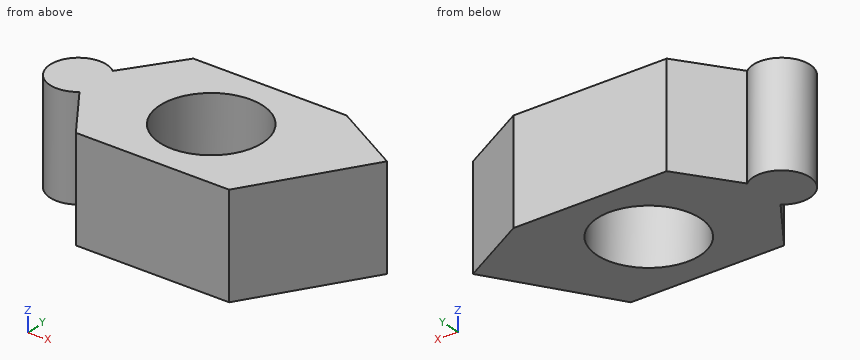
from build123d import *

# Parameters (mm, degrees)
F0_W     = 15
F0_H     = 15
F0_R     = 5
F1_DEPTH = 5
F3_DEPTH = 5
F5_DEPTH = 5


with BuildPart() as f1:
    # F0 (on Top) → F1 (new body, symmetric)
    with BuildSketch(Plane.XY):
        Rectangle(F0_W, F0_H)
        Circle(F0_R, mode=Mode.SUBTRACT)
    extrude(amount=F1_DEPTH, both=True)

    # F2 (on Top) → F3 (join, symmetric)
    with BuildSketch(Plane.XY):
        with BuildLine():
            Line((-7.5, 7.5), (-11.260282, 2.129761))
            ThreePointArc((-11.260282, 2.129761), (-15.75, 0), (-11.260282, -2.129761))
            Line((-11.260282, -2.129761), (-7.5, -7.5))
            Line((-7.5, -7.5), (-7.5, 7.5))
        make_face()
    extrude(amount=F3_DEPTH, both=True)

    # F4 (on Top) → F5 (join, symmetric)
    with BuildSketch(Plane.XY):
        Polygon((14.467447, 3.568756), (7.5, 7.5), (7.5, -7.5), align=None)
    extrude(amount=F5_DEPTH, both=True)


solid = f1.part
Geometry: final body of the model. Coordinates: model frame, mm. Coordinates: 2 decimals unless noted, no trailing zeros. Loops run counter-clockwise (first coordinate to the right, second up) from the corner with the lowest first, then second, coordinate; pieces in that order, holes last. Notation, with made-up numbers: M 9,-20.75 L 63,-20.75 A21 ccw 63,5.25 Z; hole C 28,42 d2. An arc over 180 degrees is marked long. One line per item, written item: value. Start each with the question number.
1) Cut plane D-D (x = -13). Return loops of the section in (y, z), then the cut area to 3 significant figures.
2) Pin query (flat end, axial travel): P1, Ø6, axis at x = 1, y = -4.5, coming from the +Z side; P2, Ø6, axis at y = 5, z = -0.5, coming from the +X side; P3, Ø3, axis at y = 0, z = 3, coming from the +X side; P4, Ø2, axis at x = -3, y = 1.5, coming from the +Z side. Return the tip coordinate at first contact, or that it passes through.
3) Material intervals for L1, parallel to Y at x = 0, z = -1.5; L2, parallel to X at y = 2.5, z = -0.25; L3, parallel to X at y = 3, z = 0.5, sorted ascending. Write a range as from..to.
4) Cut plane C-C (y = -1). Return loops of the section in (x, z).
5) Cut plane A-A (x = -3). Return loops of the section in (y, z), then the cut area to 3 significant figures.
6) Cut plane B-B (z = -2). Return loops of the section in (x, y).
Evaluation:
1. outline: M -2.75,-5 L 2.75,-5 L 2.75,5 L -2.75,5 Z
1. area: 55.0 mm^2
2. P1: z = 5
2. P2: x = 14.47
2. P3: x = 13.17
2. P4: through
3. L1: -7.5..-5, 5..7.5
3. L2: -14.15..-11.85, -11..-4.33, 4.33..13.79
3. L3: -10.65..-4, 4..14.11
4. outline: M -15.56,-5 L -4.9,-5 L -4.9,5 L -15.56,5 Z; M 4.9,-5 L 11.59,-5 L 11.59,5 L 4.9,5 Z
5. outline: M -7.5,-5 L -4,-5 L -4,5 L -7.5,5 Z; M 4,-5 L 7.5,-5 L 7.5,5 L 4,5 Z
5. area: 70.0 mm^2
6. outline: M -11.26,-2.13 L -7.5,-7.5 L 7.5,-7.5 L 14.47,3.57 L 7.5,7.5 L -7.5,7.5 L -11.26,2.13 A2.75 ccw long Z; hole C 0,0 d10
